Design review of the part built by this model. Coordinates are the model's own, in mm. Round coordinates to 2 decimals unless told otherwise and drop trailing zeros. Loops run counter-clockwise (first coordinate to the right, second up) from the corner with the lowest first, then second, coordinate; pieces in that order, holes last. Notation, with made-up numbers: (86.25, -29.5) -> (107.25, -29.5) arc R34 cw to (107.25, 0.5) -> close; hole circle Ø1 at (-31, 58). An arc over 180 degrees is marked (long way). Answer as CSV lines item,"result". Start each with the question number.
(1) Take a section at C-C, the plane x = -14.2. Write out the cut boundary in (y, z), and give its area (3 significant figures).
(2) Draft analysis for pull direction X (two halves, no side actions). For faces 1 (the face through (0, -17, 3.5)), 2 (the face through (-5.46, -1.05, 1.73)), 3 (the face through (15.355, -10.029, 1.774)), 4 (the face through (16.384, -3.929, 1.726)), state which applies: +X half, -X half, draft (parallel to the pull), parting line (faces both ways), or undercut.
(3) Take a section at A-A, the plane y = -9.55. Write out the cut boundary in (x, z).
(4) Take a section at D-D, the plane x = -7.5. Write out the cut boundary in (y, z), and give its area (3 significant figures).
(5) Take a section at B-B, the plane z = 0.5. Write out the cut boundary in (x, y).
(6) To check wall thickness, follow line 1 (Y direction, x = -8, z = 0.7); line 2 (X direction, y = -37.5, z = 2.9); line 3 (Y direction, x = -14.2, z = 1.15). State the ranges of each line that lie inside material, in increasing order. Write a range as from..to.
(7) For P1, Ø4.5, axis at x = 8, y = 0, coming from the +Z side, flat-tipped, find the tip position at first contact; note if it passes through.
from build123d import *

# Parameters (mm, degrees)
SKETCH1_R           = 2.75
BOSS_EXTRUDE1_DEPTH = 10
BOSS_EXTRUDE4_DEPTH = 10
SKETCH7_W           = 25
SKETCH7_H           = 2
BOSS_EXTRUDE6_DEPTH = 2
SKETCH8_R           = 1.25
CUT_EXTRUDE3_DEPTH  = 19
SKETCH9_W           = 25
SKETCH9_H           = 29.5
BOSS_EXTRUDE7_DEPTH = 10
SKETCH10_W          = 16
SKETCH10_H          = 6.5
CUT_EXTRUDE4_DEPTH  = 54


with BuildPart() as part:
    # Sketch1 → Boss-Extrude1 (new body)
    with BuildSketch(Plane.XY):
        with BuildLine():
            Line((8, 7.75), (-8, 7.75))
            ThreePointArc((-8, 7.75), (-15.75, 0), (-8, -7.75))
            Line((-8, -7.75), (8, -7.75))
            ThreePointArc((8, -7.75), (15.75, 0), (8, 7.75))
        make_face()
        with Locations((-8, 0)):
            Circle(SKETCH1_R, mode=Mode.SUBTRACT)
        with Locations((8, 0)):
            Circle(SKETCH1_R, mode=Mode.SUBTRACT)
    extrude(amount=BOSS_EXTRUDE1_DEPTH)

    # Sketch5 → Boss-Extrude4 (add)
    with BuildSketch(Plane.XY):
        Polygon((-12.5, -7.75), (-17, -7.75), (-17, -41.75), (17, -41.75), (17, -7.75), (12.5, -7.75), (12.5, -12.25), (12.5, -37.25), (-12.5, -37.25), (-12.5, -12.25), align=None)
        with BuildLine():
            ThreePointArc((-8, -7.75), (-13.480077554, -5.480077554), (-15.75, 0))
            Line((-15.75, 0), (-17, -7.75))
            Line((-17, -7.75), (-12.5, -7.75))
            Line((-12.5, -7.75), (-8, -7.75))
        make_face()
        with BuildLine():
            ThreePointArc((15.75, 0), (13.480077554, -5.480077554), (8, -7.75))
            Line((8, -7.75), (12.5, -7.75))
            Line((12.5, -7.75), (17, -7.75))
            Line((17, -7.75), (15.75, 0))
        make_face()
    extrude(amount=BOSS_EXTRUDE4_DEPTH)

    # Sketch7 → Boss-Extrude6 (add)
    with BuildSketch(Plane.XY.offset(10)):
        with Locations((0, -6.75)):
            Rectangle(SKETCH7_W, SKETCH7_H)
    extrude(amount=BOSS_EXTRUDE6_DEPTH)

    # Sketch8 → Cut-Extrude3 (cut)
    with BuildSketch(Plane.XY.offset(10)):
        with Locations((-14.2, -9.55)):
            Circle(SKETCH8_R)
        with Locations((14.2, -9.55)):
            Circle(SKETCH8_R)
        with Locations((14.2, -37.95)):
            Circle(SKETCH8_R)
        with Locations((-14.2, -37.95)):
            Circle(SKETCH8_R)
    extrude(amount=-CUT_EXTRUDE3_DEPTH, mode=Mode.SUBTRACT)

    # Sketch9 → Boss-Extrude7 (add)
    with BuildSketch(Plane(origin=(0, 0, 0), x_dir=(-1, 0, 0), z_dir=(0, 0, -1))):
        with Locations((0, -22.5)):
            Rectangle(SKETCH9_W, SKETCH9_H)
    extrude(amount=-BOSS_EXTRUDE7_DEPTH)

    # Sketch10 → Cut-Extrude4 (cut)
    with BuildSketch(Plane(origin=(0, 7.75, 0), x_dir=(1, 0, 0), z_dir=(0, 1, 0))):
        Polygon((-8, -3.5), (-17, -3.5), (-17, -13.303899359), (17, -13.303899359), (17, -3.5), (8, -3.5), (8, -10), (-8, -10), align=None)
        with Locations((0, -6.75)):
            Rectangle(SKETCH10_W, SKETCH10_H)
    extrude(amount=-CUT_EXTRUDE4_DEPTH, mode=Mode.SUBTRACT)


solid = part.part
The answers:
1,outline,"(-41.75, 0) -> (-39.2, 0) -> (-39.2, 3.5) -> (-41.75, 3.5) -> close; (-36.7, 0) -> (-10.8, 0) -> (-10.8, 3.5) -> (-36.7, 3.5) -> close; (-8.3, 0) -> (4.65, 0) -> (4.65, 3.5) -> (-8.3, 3.5) -> close"
1,area,"145 mm²"
2,face 1,"draft"
2,face 2,"undercut"
2,face 3,"undercut"
2,face 4,"+X half"
3,outline,"(-17, 0) -> (-15.45, 0) -> (-15.45, 3.5) -> (-17, 3.5) -> close; (-12.95, 0) -> (12.95, 0) -> (12.95, 3.5) -> (-12.95, 3.5) -> close; (15.45, 0) -> (17, 0) -> (17, 3.5) -> (15.45, 3.5) -> close"
4,outline,"(-41.75, 0) -> (-2.7, 0) -> (-2.7, 3.5) -> (-41.75, 3.5) -> close; (2.7, 0) -> (7.75, 0) -> (7.75, 3.5) -> (2.7, 3.5) -> close"
4,area,"154 mm²"
5,outline,"(-17, -41.75) -> (17, -41.75) -> (17, -7.75) -> (15.75, 0) arc R7.75 ccw to (8, 7.75) -> (-8, 7.75) arc R7.75 ccw to (-15.75, 0) -> (-17, -7.75) -> close; hole circle Ø2.5 at (-14.2, -37.95); hole circle Ø2.5 at (-14.2, -9.55); hole circle Ø5.5 at (-8, 0); hole circle Ø5.5 at (8, 0); hole circle Ø2.5 at (14.2, -37.95); hole circle Ø2.5 at (14.2, -9.55)"
6,line 1,"-41.75..-2.75, 2.75..7.75"
6,line 2,"-17..-15.37, -13.03..13.03, 15.37..17"
6,line 3,"-41.75..-39.2, -36.7..-10.8, -8.3..4.65"
7,P1,"through"
